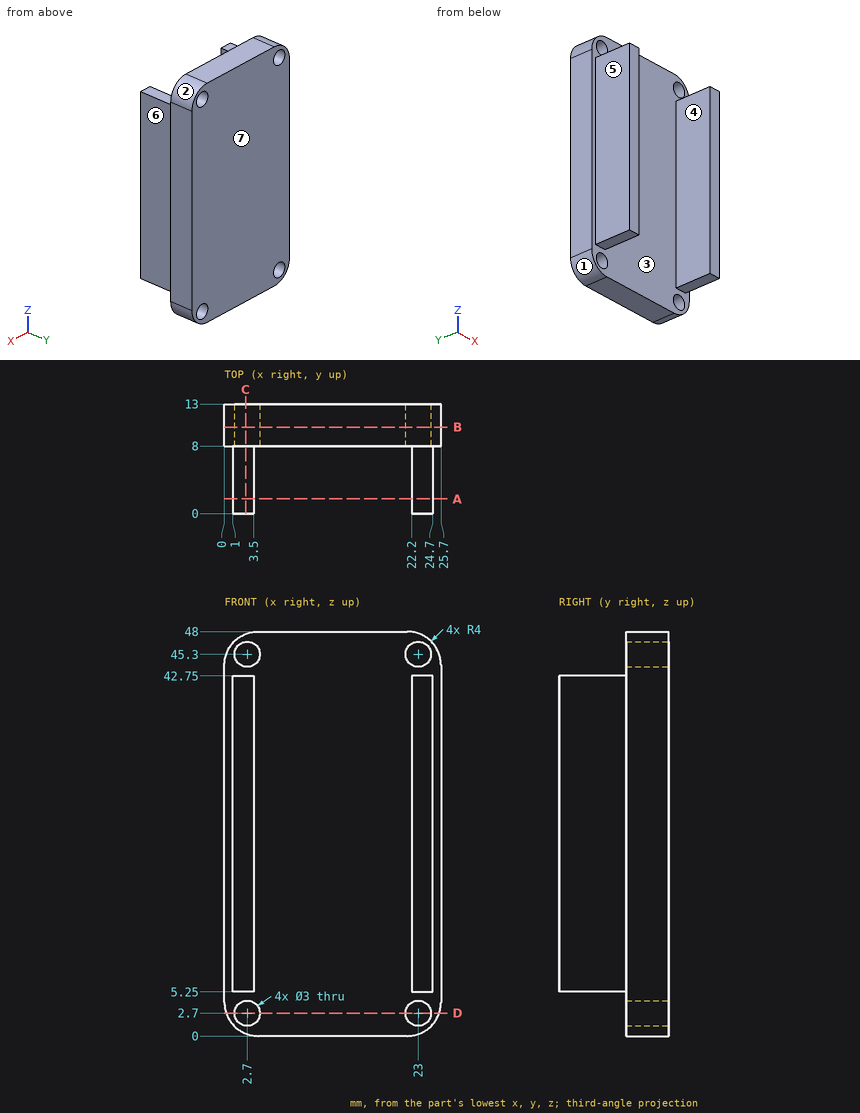
Here's the drawing with two shaded views (mm, measured from the low corner). I have some questions. A direction names the side the tool comes from. Give positions to 0.01 mm unless a question says otherwise; leave off trailing zeros. Loops run counter-clockwise (first coordinate to the right, second up) from the corner with the lowest first, then second, coordinate; pieces in that order, holes last. Notation, with made-up numbers: M -10.75,-22 L 44.25,-22 A18 ccw 44.25,-11 Z; hole C 19,41 d11. An arc over 180 degrees is marked long. Use one line per item in the form item = value. Start each with the question number.
(1) I want a section at D-D, the plane z = 2.7. Write out the boundary of the cut face in (x, y), and give its area (3 significant figures).
(2) Please list where these lines run through material, in increasing order: line 1 (X direction, y = 3, z = 29.5); line 2 (X direction, y = 11.45, z = 45.3); line 3 (Z direction, x = 2.7, y = 10.4).
(3) I'm going to push flat-ended pins straight in: P1, Ø2, axis at x = 3, y = 3.5, coming from the +Z side; P2, Ø6.5, axis at y = 2.5, z = 23.5, coming from the -X side; P3, Ø0.8, axis at x = 24, y = 5, coming from the -Z side. Where does each tip first touch, or does it pass through?
(4) Thinking about a two-plate mould opening in X: for the marked faces 1, 2, 3 and 4, which applies, released by +X, released by -X, zero draft, split by the parting line, or undercut?
(5) On a 3-axis mill with a long thin cutter (end or side, diameter ignored), from which of +Z, -Z, +X, -X, +Y, -Y can I reach the whole of each face in a straight line? I mean the marked faces 5, 6 and 7. Say none if no direction works.
(6) I want a section at C-C, the plane x = 2.5. Write out the boundary of the cut face in (y, z).
(7) I want a section at A-A, the plane y = 1.75. Write out the boundary of the cut face in (x, z).
(8) I want a section at B-B, the plane y = 10.25. Write out the boundary of the cut face in (x, z).
Worked out:
q1.outline = M 0.22,8 L 1.2,8 L 1.2,13 L 0.22,13 Z; M 4.2,8 L 21.5,8 L 21.5,13 L 4.2,13 Z; M 24.5,8 L 25.48,8 L 25.48,13 L 24.5,13 Z
q1.area = 96.3 mm²
q2.line_1 = 1 to 3.5, 22.2 to 24.7
q2.line_2 = 0.22 to 1.2, 4.2 to 21.5, 24.5 to 25.48
q2.line_3 = 0.22 to 1.2, 4.2 to 43.8, 46.8 to 47.78
q3.P1 = 42.75
q3.P2 = 1
q3.P3 = 5.25
q4.face_1 = released by -X
q4.face_2 = released by +X
q4.face_3 = undercut
q4.face_4 = undercut
q5.face_5 = +Z, -Z, -X, -Y
q5.face_6 = +Z, -Z, +X, -Y
q5.face_7 = +Z, -Z, +X, -X, +Y
q6.outline = M 0,5.25 L 8,5.25 L 8,4.19 L 13,4.19 L 13,43.81 L 8,43.81 L 8,42.75 L 0,42.75 Z; M 8,0.29 L 13,0.29 L 13,1.21 L 8,1.21 Z; M 8,46.79 L 13,46.79 L 13,47.71 L 8,47.71 Z
q7.outline = M 1,5.25 L 3.5,5.25 L 3.5,42.75 L 1,42.75 Z; M 22.2,5.25 L 24.7,5.25 L 24.7,42.75 L 22.2,42.75 Z
q8.outline = M 0,4 A4 ccw 4,0 L 21.7,0 A4 ccw 25.7,4 L 25.7,44 A4 ccw 21.7,48 L 4,48 A4 ccw 0,44 Z; hole C 2.7,2.7 d3; hole C 2.7,45.3 d3; hole C 23,2.7 d3; hole C 23,45.3 d3
